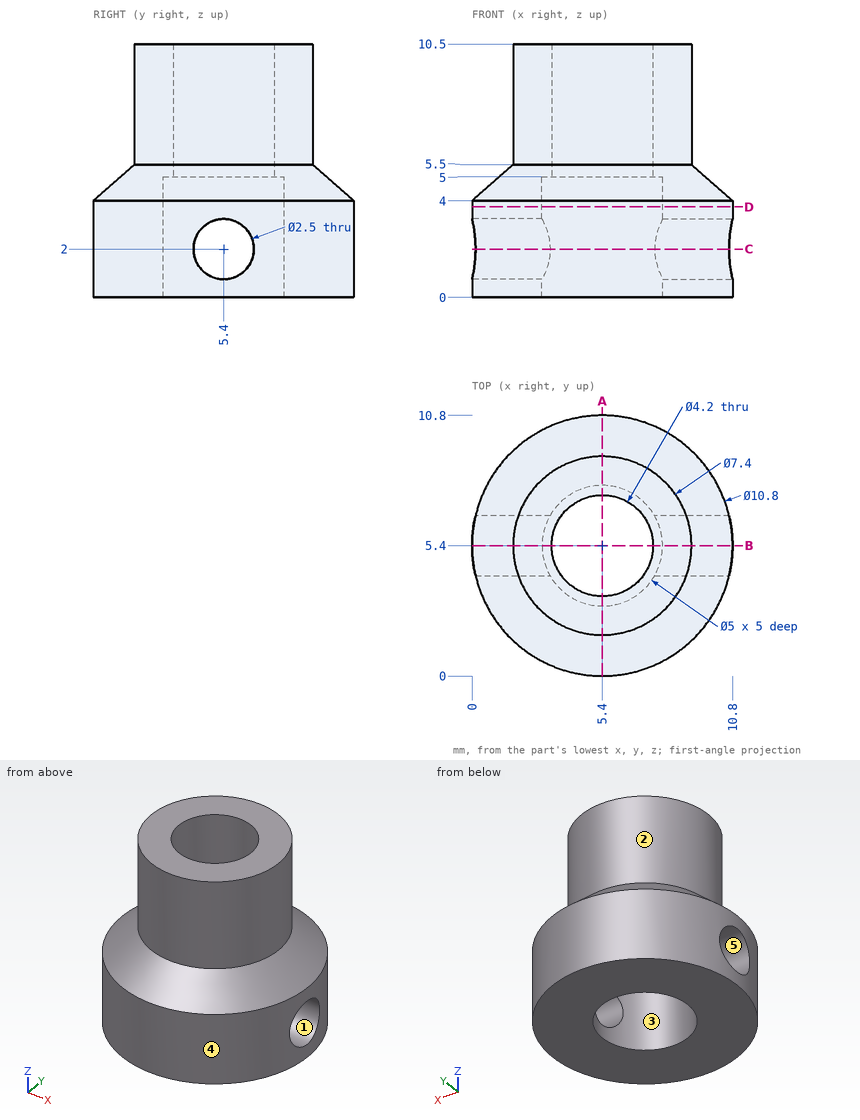
Source: three-view drawing plus pictorial views. Frame: mm from the lowest corner of the part. A direction names the side the tool comes from. Round coordinates to 2 decimals unless told otherwise and drop trailing zeros. Order: outer loops, then holes, each group sorted by start corner. A loop starts at its lowest first (then second) coordinate and runs counter-clockwise, first axis right, second up. Notation, with made-up numbers: (0, -3) - (23, -3) arc R22 cw to (23, 32) - close; hole circle Ø3 at (24.25, 24). An arc over 180 degrees is marked (long way). Use a Markdown table: item, result.
1. Material intervals for probe 1 along Y at (x, z) = (5.4, 1.65); probe 2 along Y at (x, z) = (5.4, 8.25); probe 3 along X at (y, z) = (6, 8.5), sorted ascending.
Evaluation:
| item | result |
|---|---|
| probe 1 | 0 to 2.9, 7.9 to 10.8 |
| probe 2 | 1.7 to 3.3, 7.5 to 9.1 |
| probe 3 | 1.75 to 3.39, 7.41 to 9.05 |
2. Section B-B on y = 5.4. Return the cut outline in (x, z), then the cut area to 4 significant figures.
Evaluation:
| item | result |
|---|---|
| outline | (0, 0) - (2.9, 0) - (2.9, 0.75) - (0, 0.75) - close; (0, 3.25) - (2.9, 3.25) - (2.9, 5) - (3.3, 5) - (3.3, 10.5) - (1.7, 10.5) - (1.7, 5.5) - (0, 4) - close; (7.5, 5) - (7.9, 5) - (7.9, 3.25) - (10.8, 3.25) - (10.8, 4) - (9.1, 5.5) - (9.1, 10.5) - (7.5, 10.5) - close; (7.9, 0) - (10.8, 0) - (10.8, 0.75) - (7.9, 0.75) - close |
| area | 31.25 mm^2 |
3. First-contact query: pin 1 (2 mm diameter, centred on y = 5.4, z = 2, fed in from +X); pin 2 (6 mm diameter, centred on x = 7.5, z = 8, fed in from -Y); pin 3 (4 mm diameter, centred on y = 9.5, z = 4.5, fed in from +X); pin 4 (6 mm diameter, centred on x = 8, z = 7.5, fed in from -Y). Flat tips, straight axial feed; report the tip coordinate or a pass-through.
Evaluation:
| item | result |
|---|---|
| pin 1 | through |
| pin 2 | y = 1.47 |
| pin 3 | x = 10.35 |
| pin 4 | y = 1.04 |
4. Access query for the marked faces 1 and 2. Directions: +Z, -Z, +X, -X, +Y, -Y. A direction counts if a zero-diameter tool reaches every point of the face in a straight line with its end or side. Return the directions, or none.
Evaluation:
| item | result |
|---|---|
| face 1 | +X, -X |
| face 2 | +Z |
5. Section C-C on z = 2. Return the cut outline in (x, y), then the cut area to 3 significant figures.
Evaluation:
| item | result |
|---|---|
| outline | (0.15, 4.15) arc R5.4 ccw to (10.65, 4.15) - (7.57, 4.15) arc R2.5 cw to (3.23, 4.15) - close; (0.15, 6.65) - (3.23, 6.65) arc R2.5 cw to (7.57, 6.65) - (10.65, 6.65) arc R5.4 ccw to start |
| area | 57.2 mm^2 |
6. Section A-A on x = 5.4. Return the cut outline in (y, z), then the cut area to 4 significant figures.
Evaluation:
| item | result |
|---|---|
| outline | (0, 0) - (2.9, 0) - (2.9, 5) - (3.3, 5) - (3.3, 10.5) - (1.7, 10.5) - (1.7, 5.5) - (0, 4) - close; (7.5, 5) - (7.9, 5) - (7.9, 0) - (10.8, 0) - (10.8, 4) - (9.1, 5.5) - (9.1, 10.5) - (7.5, 10.5) - close |
| area | 45.75 mm^2 |
7. Section D-D on z = 3.75. Return the cut outline in (x, y).
Evaluation:
| item | result |
|---|---|
| outline | circle Ø10.8 at (5.4, 5.4); hole circle Ø5 at (5.4, 5.4) |
8. Mould query, pull axis X, two halves, no side actions, for the marked faces 3, 4 and 5. Classes: +X half, -X half, draft (parallel to the pull), parting line (faces both ways), or undercut.
Evaluation:
| item | result |
|---|---|
| face 3 | undercut |
| face 4 | parting line |
| face 5 | draft |
